Work out the finished part from the listing and answer in its coordinate system (mm). Face numbers are marked on the shaded views. Coordinates: 2 decimals unless noted, no trailing zeros. Write each loop counter-clockwise with the first axis right and the second up, starting at its lowest first coordinate (ties: lowest second). Pieces come first, ordered by that corner, then holes. Notation, with made-up numbers: (88.5, 39) -> (141.5, 39) arc R21 ccw to (141.5, 77) -> close; hole circle Ø4 at (57, -13.75). An arc over 180 degrees is marked (long way). Write each question's results on one line, items separated by ' | '. Start each with the question number.
from build123d import *
from build123d.topology import SkipClean

# Parameters (mm, degrees)
SKETCH1_R           = 1.25
BOSS_EXTRUDE1_DEPTH = 2.5
BOSS_EXTRUDE2_START = 23.5
BOSS_EXTRUDE2_DEPTH = 26
BOSS_EXTRUDE3_START = 23.5
SKETCH1_4_R         = 1.25
BOSS_EXTRUDE3_DEPTH = 3


with BuildPart() as part:
    # Sketch1 → Boss-Extrude1 (new body)
    with BuildSketch(Plane(origin=(0, 0, 0), x_dir=(1, 0, 0), z_dir=(0, 1, 0))):
        with BuildLine():
            Line((-50.40491586, 135.957141986), (-31.25, 89.71308433))
            Line((-31.25, 89.71308433), (31.25, 89.71308433))
            Line((31.25, 89.71308433), (50.40491586, 135.957141986))
            ThreePointArc((50.40491586, 135.957141986), (0, 145), (-50.40491586, 135.957141986))
        make_face()
        with Locations(Location((-2.5, 91.868329805, 0), (0, 0, 270))):
            Circle(SKETCH1_R, mode=Mode.SUBTRACT)
        with Locations(Location((2.5, 91.868329805, 0), (0, 0, 270))):
            Circle(SKETCH1_R, mode=Mode.SUBTRACT)
        with BuildLine():
            Line((-26.870747539, 121.475518488), (-24.957330377, 116.856120826))
            ThreePointArc((-24.957330377, 116.856120826), (-24.727253788, 116.604473302), (-24.389349959, 116.558836529))
            ThreePointArc((-24.389349959, 116.558836529), (0, 119.174853647), (24.389349959, 116.558836529))
            ThreePointArc((24.389349959, 116.558836529), (24.727253788, 116.604473302), (24.957330377, 116.856120826))
            Line((24.957330377, 116.856120826), (26.870747539, 121.475518488))
            ThreePointArc((26.870747539, 121.475518488), (26.851801477, 121.898714852), (26.514867242, 122.155482133))
            ThreePointArc((26.514867242, 122.155482133), (0, 125), (-26.514867242, 122.155482133))
            ThreePointArc((-26.514867242, 122.155482133), (-26.851801477, 121.898714852), (-26.870747539, 121.475518488))
        make_face(mode=Mode.SUBTRACT)
    extrude(amount=-BOSS_EXTRUDE1_DEPTH)

    # Sketch1<3> → Boss-Extrude2 (add)
    with SkipClean():  # the faces are left unmerged after this step: merging them gives an invalid solid
        with BuildSketch(Plane(origin=(0, 0, 0), x_dir=(1, 0, 0), z_dir=(0, 1, 0)).offset(BOSS_EXTRUDE2_START)):
            with BuildLine():
                ThreePointArc((-26.780015914, 123.377036954), (-27.959285739, 122.478351471), (-28.025596955, 120.997164198))
                Line((-28.025596955, 120.997164198), (-26.112179793, 116.377766535))
                ThreePointArc((-26.112179793, 116.377766535), (-25.467638519, 115.59239072), (-24.495390611, 115.297462542))
                Line((-24.495390611, 115.297462542), (24.495390611, 115.297462542))
                ThreePointArc((24.495390611, 115.297462542), (25.467638519, 115.59239072), (26.112179793, 116.377766535))
                Line((26.112179793, 116.377766535), (28.025596955, 120.997164198))
                ThreePointArc((28.025596955, 120.997164198), (27.959285739, 122.478351471), (26.780015914, 123.377036954))
                ThreePointArc((26.780015914, 123.377036954), (0, 126.25), (-26.780015914, 123.377036954))
            make_face()
            with BuildLine():
                Line((-24.957330377, 116.856120826), (-26.870747539, 121.475518488))
                ThreePointArc((-26.870747539, 121.475518488), (-26.851801477, 121.898714852), (-26.514867242, 122.155482133))
                ThreePointArc((-26.514867242, 122.155482133), (0, 125), (26.514867242, 122.155482133))
                ThreePointArc((26.514867242, 122.155482133), (26.851801477, 121.898714852), (26.870747539, 121.475518488))
                Line((26.870747539, 121.475518488), (24.957330377, 116.856120826))
                ThreePointArc((24.957330377, 116.856120826), (24.727253788, 116.604473302), (24.389349959, 116.558836529))
                ThreePointArc((24.389349959, 116.558836529), (0, 119.174853647), (-24.389349959, 116.558836529))
                ThreePointArc((-24.389349959, 116.558836529), (-24.727253788, 116.604473302), (-24.957330377, 116.856120826))
            make_face(mode=Mode.SUBTRACT)
        extrude(amount=-BOSS_EXTRUDE2_DEPTH)
    add(part.part.scale(1), mode=Mode.REPLACE)  # the faces are merged on a copy

    # Sketch1<4> → Boss-Extrude3 (add)
    # profile 1 of 2: a face of its own
    with BuildSketch(Plane(origin=(0, 0, 0), x_dir=(1, 0, 0), z_dir=(0, 1, 0)).offset(BOSS_EXTRUDE3_START)):
        with BuildLine():
            ThreePointArc((-50.40491586, 135.957141986), (0, 145), (50.40491586, 135.957141986))
            Line((50.40491586, 135.957141986), (31.25, 89.71308433))
            Line((31.25, 89.71308433), (-31.25, 89.71308433))
            Line((-31.25, 89.71308433), (-50.40491586, 135.957141986))
        make_face()
        with Locations(Location((2.5, 91.868329805, 0), (0, 0, 270))):
            Circle(SKETCH1_4_R, mode=Mode.SUBTRACT)
        with Locations(Location((-2.5, 91.868329805, 0), (0, 0, 270))):
            Circle(SKETCH1_4_R, mode=Mode.SUBTRACT)
        with BuildLine():
            Line((-28.025596955, 120.997164198), (-26.112179793, 116.377766535))
            ThreePointArc((-26.112179793, 116.377766535), (-25.467638519, 115.59239072), (-24.495390611, 115.297462542))
            Line((-24.495390611, 115.297462542), (24.495390611, 115.297462542))
            ThreePointArc((24.495390611, 115.297462542), (25.467638519, 115.59239072), (26.112179793, 116.377766535))
            Line((26.112179793, 116.377766535), (28.025596955, 120.997164198))
            ThreePointArc((28.025596955, 120.997164198), (27.959285739, 122.478351471), (26.780015914, 123.377036954))
            ThreePointArc((26.780015914, 123.377036954), (0, 126.25), (-26.780015914, 123.377036954))
            ThreePointArc((-26.780015914, 123.377036954), (-27.959285739, 122.478351471), (-28.025596955, 120.997164198))
        make_face(mode=Mode.SUBTRACT)
    # profile 2 of 2: a face of its own
    with BuildSketch(Plane(origin=(0, 0, 0), x_dir=(1, 0, 0), z_dir=(0, 1, 0)).offset(BOSS_EXTRUDE3_START)):
        with BuildLine():
            ThreePointArc((-28.025596955, 120.997164198), (-27.959285739, 122.478351471), (-26.780015914, 123.377036954))
            ThreePointArc((-26.780015914, 123.377036954), (0, 126.25), (26.780015914, 123.377036954))
            ThreePointArc((26.780015914, 123.377036954), (27.959285739, 122.478351471), (28.025596955, 120.997164198))
            Line((28.025596955, 120.997164198), (26.112179793, 116.377766535))
            ThreePointArc((26.112179793, 116.377766535), (25.467638519, 115.59239072), (24.495390611, 115.297462542))
            Line((24.495390611, 115.297462542), (-24.495390611, 115.297462542))
            ThreePointArc((-24.495390611, 115.297462542), (-25.467638519, 115.59239072), (-26.112179793, 116.377766535))
            Line((-26.112179793, 116.377766535), (-28.025596955, 120.997164198))
        make_face()
        with BuildLine():
            Line((26.870747539, 121.475518488), (24.957330377, 116.856120826))
            ThreePointArc((24.957330377, 116.856120826), (24.727253788, 116.604473302), (24.389349959, 116.558836529))
            ThreePointArc((24.389349959, 116.558836529), (0, 119.174853647), (-24.389349959, 116.558836529))
            ThreePointArc((-24.389349959, 116.558836529), (-24.727253788, 116.604473302), (-24.957330377, 116.856120826))
            Line((-24.957330377, 116.856120826), (-26.870747539, 121.475518488))
            ThreePointArc((-26.870747539, 121.475518488), (-26.851801477, 121.898714852), (-26.514867242, 122.155482133))
            ThreePointArc((-26.514867242, 122.155482133), (0, 125), (26.514867242, 122.155482133))
            ThreePointArc((26.514867242, 122.155482133), (26.851801477, 121.898714852), (26.870747539, 121.475518488))
        make_face(mode=Mode.SUBTRACT)
    extrude(amount=-BOSS_EXTRUDE3_DEPTH)


solid = part.part
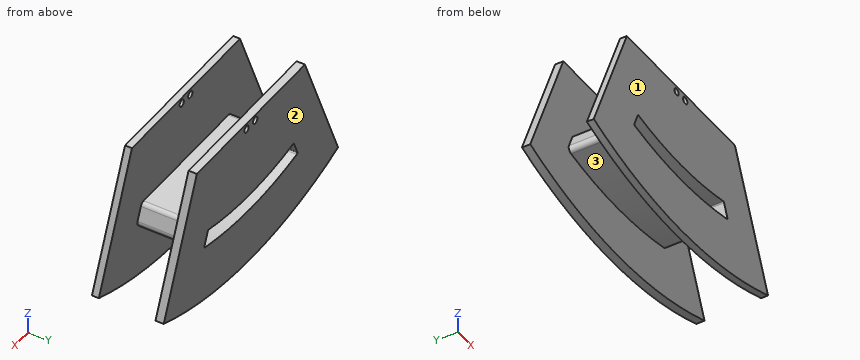
1. Find section A-A on y = 15. Give the vertices of the cut face in (x, z), and give its area (3 significant figures).
2. Find section D-D on x = 2.5. Give the vertices of the cut face in (y, z) (3 decimals), and give its area (3 significant figures).
3. Given pin 1 Ø4 at (x, z) = (2.5, -91.87) entering from -Y; pin 2 Ø1.5 at (x, y) = (24.5, 6.5) entering from -Z, each flat-ended and moving along its own axis, determine where each tip first touches the part or whether it passes through.
4. Find the intervals of material crossed by L1, parallel to Y at x = 36, z = -122.5; L2, parallel to Z at x = -23, y = 11; L3, parallel to Z at x = 8, y = 5.5, in increasing order.
5. Find section C-C on z = -94.5. Give the vertices of the cut face in (x, y).
6. Determine the mould class of the marked faces 1, 2 and 3 for opening direction Y: pulls with the +Y half, pulls with the -Y half, needs draft (parallel to the pull), parting line crosses it, or undercut.
7. Find section B-B on x = -18. Give the vertices of the cut face in (y, z), and give its area (3 significant figures).
Ans:
1) outline: (-28.03, -121) arc R1.75 ccw to (-26.78, -123.38) arc R126.25 ccw to (26.78, -123.38) arc R1.75 ccw to (28.03, -121) -> (26.11, -116.38) arc R1.75 ccw to (24.5, -115.3) -> (-24.5, -115.3) arc R1.75 ccw to (-26.11, -116.38) -> close; hole (-26.87, -121.48) arc R0.5 ccw to (-26.51, -122.16) arc R125 ccw to (26.51, -122.16) arc R0.5 ccw to (26.87, -121.48) -> (24.96, -116.86) arc R0.5 ccw to (24.39, -116.56) arc R115 cw to (-24.39, -116.56) arc R0.5 ccw to (-24.96, -116.86) -> close | area: 235 mm²
2) outline: (-2.5, -144.978) -> (0, -144.978) -> (0, -126.225) -> (20.5, -126.225) -> (20.5, -144.978) -> (23.5, -144.978) -> (23.5, -124.975) -> (-2.5, -124.975) -> close; (-2.5, -119.148) -> (23.5, -119.148) -> (23.5, -93.118) -> (20.5, -93.118) -> (20.5, -115.297) -> (0, -115.297) -> (0, -93.118) -> (-2.5, -93.118) -> close; (-2.5, -90.618) -> (0, -90.618) -> (0, -89.713) -> (-2.5, -89.713) -> close; (20.5, -90.618) -> (23.5, -90.618) -> (23.5, -89.713) -> (20.5, -89.713) -> close | area: 363 mm²
3) pin 1: stops at y = -2.5 | pin 2: stops at z = -124
4) L1: y = -2.5 to 0, 20.5 to 23.5 | L2: z = -124.14 to -122.87, -116.85 to -115.3 | L3: z = -126 to -124.74, -118.9 to -115.3
5) outline: (-33.23, -2.5) -> (33.23, -2.5) -> (33.23, 0) -> (-33.23, 0) -> close; (-33.23, 20.5) -> (33.23, 20.5) -> (33.23, 23.5) -> (-33.23, 23.5) -> close
6) face 1: pulls with the -Y half | face 2: pulls with the +Y half | face 3: undercut
7) outline: (-2.5, -143.88) -> (0, -143.88) -> (0, -124.96) -> (20.5, -124.96) -> (20.5, -143.88) -> (23.5, -143.88) -> (23.5, -123.7) -> (-2.5, -123.7) -> close; (-2.5, -117.76) -> (23.5, -117.76) -> (23.5, -89.71) -> (20.5, -89.71) -> (20.5, -115.3) -> (0, -115.3) -> (0, -89.71) -> (-2.5, -89.71) -> close | area: 342 mm²
